Here's how the part is built. I have some questions about the finished solid (model axes, mm). A direction names the side the tool comes from. Round coordinates to 2 decimals unless told otherwise and drop trailing zeros. Loops run counter-clockwise (first coordinate to the right, second up) from the corner with the lowest first, then second, coordinate; pieces in that order, holes last. Notation, with made-up numbers: M 48.25,-36 L 93.25,-36 A19 ccw 93.25,-7 Z; hole C 89.5,70 d6. An arc over 180 degrees is marked long. Answer as CSV lines item,"result".
```python
from build123d import *

# Parameters (mm, degrees)
SKETCH1_R           = 30
BOSS_EXTRUDE1_DEPTH = 5
SKETCH2_W           = 60
SKETCH2_H           = 40
BOSS_EXTRUDE2_DEPTH = 5
SKETCH3_R           = 1.45
CUT_EXTRUDE1_DEPTH  = 5
SKETCH4_R           = 1.45
BOSS_EXTRUDE3_DEPTH = 4
SKETCH5_W           = 22
SKETCH5_H           = 11.5
BOSS_EXTRUDE4_DEPTH = 108.5


with BuildPart() as part:
    # Sketch1 → Boss-Extrude1 (new body)
    with BuildSketch(Plane.XY.offset(384.5)):
        with Locations((300, 300)):
            Circle(SKETCH1_R)
    extrude(amount=BOSS_EXTRUDE1_DEPTH)

    # Sketch2 → Boss-Extrude2 (add)
    with BuildSketch(Plane.XY.offset(384.5)):
        with Locations((300, 320)):
            Rectangle(SKETCH2_W, SKETCH2_H)
    extrude(amount=BOSS_EXTRUDE2_DEPTH)

    # Sketch3 → Cut-Extrude1 (cut)
    with BuildSketch(Plane.XY.offset(384.5)):
        with Locations((286.774831823, 318.202882373)):
            Circle(SKETCH3_R)
        with Locations((278.601228383, 293.047117627)):
            Circle(SKETCH3_R)
        with Locations((300, 277.5)):
            Circle(SKETCH3_R)
        with Locations((321.398771617, 293.047117627)):
            Circle(SKETCH3_R)
        with Locations((313.225168177, 318.202882373)):
            Circle(SKETCH3_R)
        with BuildLine():
            Line((292.928932188, 292.928932188), (300, 285.857864376))
            Line((300, 285.857864376), (307.071067812, 292.928932188))
            ThreePointArc((307.071067812, 292.928932188), (300, 310), (292.928932188, 292.928932188))
        make_face()
    extrude(amount=CUT_EXTRUDE1_DEPTH, mode=Mode.SUBTRACT)



with BuildPart() as body_2:
    # Sketch4 → Boss-Extrude3 (new body)
    with BuildSketch(Plane.XY.offset(276)):
        Polygon((289, 340), (311, 340), (311, 334), (330, 315), (330, 270), (311, 270), (311, 260), (289, 260), (289, 270), (270, 270), (270, 315), (289, 334), align=None)
        with Locations((286.774831823, 318.202882373)):
            Circle(SKETCH4_R, mode=Mode.SUBTRACT)
        with Locations((278.601228383, 293.047117627)):
            Circle(SKETCH4_R, mode=Mode.SUBTRACT)
        with Locations((300, 277.5)):
            Circle(SKETCH4_R, mode=Mode.SUBTRACT)
        with Locations((321.398771617, 293.047117627)):
            Circle(SKETCH4_R, mode=Mode.SUBTRACT)
        with Locations((313.225168177, 318.202882373)):
            Circle(SKETCH4_R, mode=Mode.SUBTRACT)
        with BuildLine():
            Line((292.928932188, 292.928932188), (300, 285.857864376))
            Line((300, 285.857864376), (307.071067812, 292.928932188))
            ThreePointArc((307.071067812, 292.928932188), (300, 310), (292.928932188, 292.928932188))
        make_face(mode=Mode.SUBTRACT)
    extrude(amount=BOSS_EXTRUDE3_DEPTH)


with BuildPart() as part_1:
    add(part.part)

    add(body_2.part)  # Boss-Extrude4 merges body 2
    # Sketch5 → Boss-Extrude4 (add)
    with BuildSketch(Plane.XY.offset(276)):
        with Locations((300, 334.25)):
            Rectangle(SKETCH5_W, SKETCH5_H)
    extrude(amount=BOSS_EXTRUDE4_DEPTH)


solid = part_1.part
```
1. We'd pull the mould along Z, two halves only. Please class faces 1 (the flat face through (320, 325, 278)), 2 (the flat face through (293.8, 291.7, 276)), 3 (the flat face through (311, 334, 329)): pulls with the +Z half, pulls with the -Z half, needs draft (parallel to the pull), parting line crosses it, or undercut.
Evaluation:
face 1,"needs draft"
face 2,"pulls with the -Z half"
face 3,"undercut"
2. I want a section at C-C, the plane x = 297. Please give me the cut outline in (y, z).
Evaluation:
outline,"M 260,276 L 288.86,276 L 288.86,280 L 260,280 Z; M 270.15,384.5 L 288.86,384.5 L 288.86,389.5 L 270.15,389.5 Z; M 309.54,276 L 340,276 L 340,389.5 L 309.54,389.5 L 309.54,384.5 L 328.5,384.5 L 328.5,280 L 309.54,280 Z"
3. If I drill on line 1 (Y direction, x = 300, z = 386); line 2 (Z direction, x = 291, y = 309.5); line 3 (Z direction, x = 318, y = 272), over which ranges is the centre line in solid material (lowest first)? Write a range as [from, to].
Evaluation:
line 1,"y = [270, 276.05], [278.95, 285.86], [310, 340]"
line 2,"z = [276, 280], [384.5, 389.5]"
line 3,"z = [276, 280]"
4. I want a section at B-B, the plane y = 324. Please give me the cut outline in (x, z), and give its area (3 significant figures).
Evaluation:
outline,"M 270,384.5 L 330,384.5 L 330,389.5 L 270,389.5 Z; M 279,276 L 321,276 L 321,280 L 279,280 Z"
area,"468 mm²"
5. For P1, Ø1.7, axis at x = 286.77, y = 318.2, coming from the -Z side; P2, Ø3, axis at x = 284.5, y = 269.5, coming from the +Z side; P3, Ø3, axis at x = 299, z = 359.5, coming from the -Y side; P4, Ø9, axis at y = 336.5, z = 329, coming from the +X side, each with a flat end and sliding along its axis, tell me the tip position at first contact or that it passes through.
Evaluation:
P1,"passes through"
P2,"stops at z = 280"
P3,"stops at y = 328.5"
P4,"stops at x = 311"
6. I want a section at A-A, the plane x = 282. Please give me the cut outline in (y, z), and give its area (3 significant figures).
Evaluation:
outline,"M 270,276 L 327,276 L 327,280 L 270,280 Z; M 276,384.5 L 340,384.5 L 340,389.5 L 276,389.5 Z"
area,"548 mm²"
7. Which directions (+Z, -Z, +X, -X, +Y, -Y) give clear straight access to the entire face, cutting with the end or side of a thin tool? Please do faces 4 (the flat face through (300, 260, 278)), 5 (the flat face through (270, 292, 278)), 6 (the cylindrical face through (299.34, 270.007, 386.965)), 7 (the flat face through (303.486, 289.344, 277.972)), 8 (the flat face through (289, 265, 278)).
Evaluation:
face 4,"+Z, -Z, +X, -X, -Y"
face 5,"+Z, -Z, -X, +Y, -Y"
face 6,"+Z, -Y"
face 7,"+Z, -Z"
face 8,"+Z, -Z, -X, -Y"
8. I want a section at D-D, the plane y = 277.5. Please give me the cut outline in (x, z), and give its area (3 significant figures).
Evaluation:
outline,"M 270,276 L 298.55,276 L 298.55,280 L 270,280 Z; M 280.16,384.5 L 298.55,384.5 L 298.55,389.5 L 280.16,389.5 Z; M 301.45,276 L 330,276 L 330,280 L 301.45,280 Z; M 301.45,384.5 L 319.84,384.5 L 319.84,389.5 L 301.45,389.5 Z"
area,"412 mm²"
